For this review, use the dimensioned drawing (mm, ordinates from the lowest corner) and the shaded views. Coordinates: 2 decimals unless noted, no trailing zeros. Loops run counter-clockwise (first coordinate to the right, second up) from the corner with the lowest first, then second, coordinate; pieces in that order, holes last. Notation, with made-up numbers: M 25,-8.75 L 50,-8.75 A24 ccw 50,2.25 Z; hole C 70,-10.75 d6. An arc over 180 degrees is marked long. One line per item, written item: value.
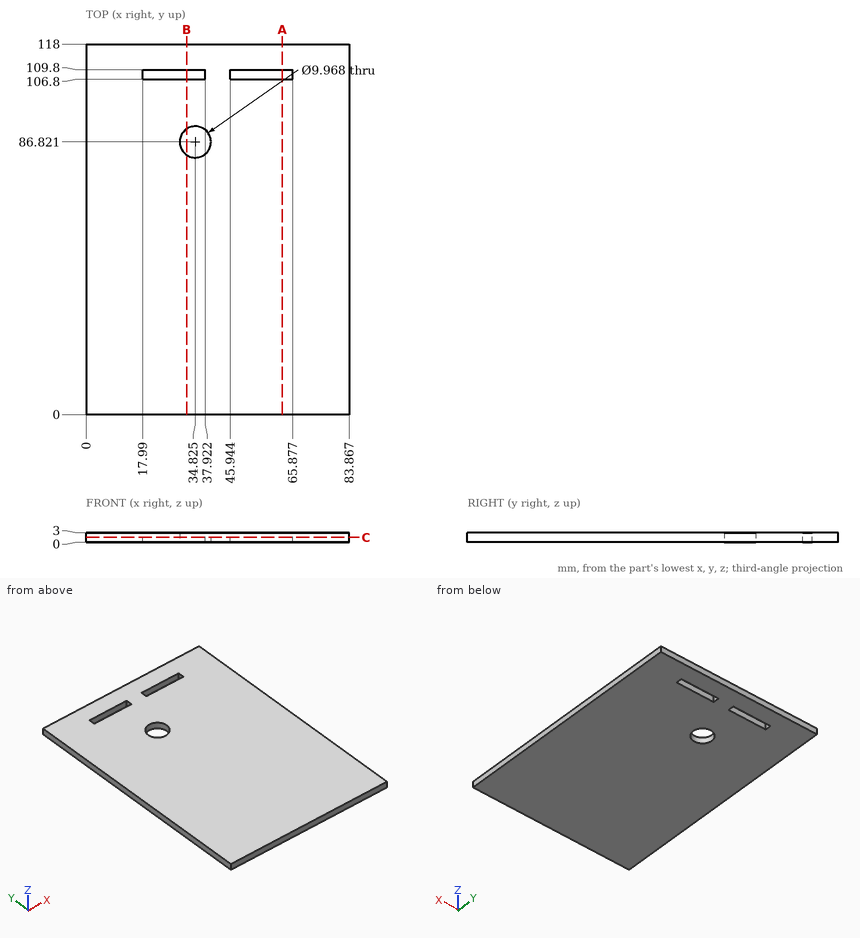
(1) Add section A-A on x = 62.5. State the section outline as (y, z) points, then the cut area to 3 significant figures.
Checks:
outline: M 0,0 L 106.8,0 L 106.8,3 L 0,3 Z; M 109.8,0 L 118,0 L 118,3 L 109.8,3 Z
area: 345 mm^2
(2) Insertion check: pin 1 Ø6 at (x, y) = (34.83, 86.82) entering from -Z. The pin has a flat end and moves straight along its axis. Give the tip position at first contact, or say it passes through.
Checks:
pin 1: through
(3) Add section C-C on z = 1.5. State the section outline as (x, y) points (1 decimal).
Checks:
outline: M 0,0 L 83.9,0 L 83.9,118 L 0,118 Z; hole M 18,106.8 L 37.9,106.8 L 37.9,109.8 L 18,109.8 Z; hole C 34.8,86.8 d10; hole M 45.9,106.8 L 65.9,106.8 L 65.9,109.8 L 45.9,109.8 Z
(4) To check wall thickness, follow L1, parallel to Y at x = 35, z = 2.85; L2, parallel to Y at x = 47, z = 1.7; L3, parallel to X at y = 85, z = 0.75 (1 decimal). State the ranges of each line that lie inside material, in increasing order. Write a range as [from, to].
Checks:
L1: [0, 81.84], [91.8, 106.8], [109.8, 118]
L2: [0, 106.8], [109.8, 118]
L3: [0, 30.2], [39.5, 83.9]
(5) Add section B-B on x = 32. State the section outline as (y, z) points (1 decimal).
Checks:
outline: M 0,0 L 82.7,0 L 82.7,3 L 0,3 Z; M 90.9,0 L 106.8,0 L 106.8,3 L 90.9,3 Z; M 109.8,0 L 118,0 L 118,3 L 109.8,3 Z
